```python
from build123d import *

# Parameters (mm, degrees)
SKETCH_1_W          = 40
SKETCH_1_H          = 14
EXTRUDE_1_DEPTH     = 40
SKETCH_6_W          = 36
SKETCH_6_H          = 10
CUT_EXTRUDE_2_DEPTH = 41
SKETCH_15_OUTSIDE_W = 53.656
SKETCH_15_OUTSIDE_H = 27.656
CUT_EXTRUDE_5_DEPTH = 41
SKETCH_16_W         = 50
SKETCH_16_H         = 24
EXTRUDE_2_DEPTH     = 1
SKETCH_17_W         = 50
SKETCH_17_H         = 24
EXTRUDE_3_DEPTH     = 1
SKETCH_18_W         = 36
SKETCH_18_H         = 10
CUT_EXTRUDE_6_DEPTH = 1


with BuildPart() as part:
    # 草图1 → 凸台-拉伸1 (new body)
    with BuildSketch(Plane(origin=(0, 0, 0), x_dir=(1, 0, 0), z_dir=(0, 1, 0))):
        with Locations((20, 7)):
            Rectangle(SKETCH_1_W, SKETCH_1_H)
    extrude(amount=EXTRUDE_1_DEPTH)

    # 草图6 → 切除-拉伸2 (cut, through all)
    with BuildSketch(Plane(origin=(0, 40, 0), x_dir=(1, 0, 0), z_dir=(0, 1, 0))):
        with Locations((20, 7)):
            Rectangle(SKETCH_6_W, SKETCH_6_H)
    extrude(amount=-CUT_EXTRUDE_2_DEPTH, mode=Mode.SUBTRACT)

    # 草图15 outside → 切除-拉伸5 (cut, through all)
    with BuildSketch(Plane.XZ):
        with Locations((20, -7)):
            Rectangle(SKETCH_15_OUTSIDE_W, SKETCH_15_OUTSIDE_H)
        with BuildLine():
            Line((2, -14), (38, -14))
            ThreePointArc((38, -14), (39.414213562, -13.414213562), (40, -12))
            Line((40, -12), (40, -2))
            ThreePointArc((40, -2), (39.414213562, -0.585786438), (38, 0))
            Line((38, 0), (2, 0))
            ThreePointArc((2, 0), (0.585786438, -0.585786438), (0, -2))
            Line((0, -2), (0, -12))
            ThreePointArc((0, -12), (0.585786438, -13.414213562), (2, -14))
        make_face(mode=Mode.SUBTRACT)
    extrude(amount=-CUT_EXTRUDE_5_DEPTH, mode=Mode.SUBTRACT)

    # 草图16 → 凸台-拉伸2 (add)
    with BuildSketch(Plane(origin=(0, 40, 0), x_dir=(1, 0, 0), z_dir=(0, 1, 0))):
        with Locations((20, 7)):
            Rectangle(SKETCH_16_W, SKETCH_16_H)
    extrude(amount=EXTRUDE_2_DEPTH)

    # 草图17 → 凸台-拉伸3 (add)
    with BuildSketch(Plane.XZ):
        with Locations((20, -7)):
            Rectangle(SKETCH_17_W, SKETCH_17_H)
    extrude(amount=EXTRUDE_3_DEPTH)

    # 草图18 → 切除-拉伸6 (cut)
    with BuildSketch(Plane(origin=(0, -1, 0), x_dir=(-1, 0, 0), z_dir=(0, -1, 0))):
        with Locations((-20, 7)):
            Rectangle(SKETCH_18_W, SKETCH_18_H)
    extrude(amount=-CUT_EXTRUDE_6_DEPTH, mode=Mode.SUBTRACT)


solid = part.part
```
Can you work these out from the model? Positions are in its coordinate system, mm. A direction names the side the tool comes from. Coordinates: 2 decimals unless noted, no trailing zeros. Loops run counter-clockwise (first coordinate to the right, second up) from the corner with the lowest first, then second, coordinate; pieces in that order, holes last. Notation, with made-up numbers: (53.25, 51.5) - (78.25, 51.5) arc R12 ccw to (78.25, 71.5) - close; hole circle Ø8 at (49, 6). An arc over 180 degrees is marked (long way). Use a Markdown table: item, result.
Item 1: I want a section at D-D on x = 29.5. Please give me the cut outline in (y, z).
Numbers:
| item | result |
|---|---|
| outline | (-1, -19) - (0, -19) - (0, -14) - (40, -14) - (40, -19) - (41, -19) - (41, 5) - (40, 5) - (40, 0) - (0, 0) - (0, 5) - (-1, 5) - (-1, -2) - (40, -2) - (40, -12) - (-1, -12) - close |
Item 2: I want a section at C-C on z = -10.5. Please give me the cut outline in (x, y).
Numbers:
| item | result |
|---|---|
| outline | (-5, -1) - (2, -1) - (2, 40) - (38, 40) - (38, -1) - (45, -1) - (45, 0) - (40, 0) - (40, 40) - (45, 40) - (45, 41) - (-5, 41) - (-5, 40) - (0, 40) - (0, 0) - (-5, 0) - close |
Item 3: I want a section at B-B on y = 33. Please give me the cut outline in (x, z).
Numbers:
| item | result |
|---|---|
| outline | (0, -12) arc R2 ccw to (2, -14) - (38, -14) arc R2 ccw to (40, -12) - (40, -2) arc R2 ccw to (38, 0) - (2, 0) arc R2 ccw to (0, -2) - close; hole (2, -12) - (38, -12) - (38, -2) - (2, -2) - close |
Item 4: We'd pull the mould along Z, two halves only. Please class faces 6 (the face through (0.57, 19.72, -13.4)), 7 (the face through (40, 20, -7)), 8 (the face through (38, 19, -7)): released by +Z, released by -Z, zero draft, split by the parting line, or undercut.
Numbers:
| item | result |
|---|---|
| face 6 | released by -Z |
| face 7 | zero draft |
| face 8 | undercut |
Item 5: For faces 1 (the face through (0.6, 19.72, -0.57)), 2 (the face through (39.4, 19.72, -13.43)), 3 (the face through (20, 19, -2)), 4 (the face through (0, 20, -7)), 5 (the face through (20, 20, 0)), which set-ups out of +Z, -Z, +X, -X, +Y, -Y let a thin tool reach every point of the face, with its end or its side?
Numbers:
| item | result |
|---|---|
| face 1 | +Z, -X |
| face 2 | -Z, +X |
| face 3 | -Y |
| face 4 | +Z, -Z, -X |
| face 5 | +Z, +X, -X |
Item 6: I want a section at A-A on z = -16.75. Please give me the cut outline in (x, y), and give its area (3 significant figures).
Numbers:
| item | result |
|---|---|
| outline | (-5, -1) - (45, -1) - (45, 0) - (-5, 0) - close; (-5, 40) - (45, 40) - (45, 41) - (-5, 41) - close |
| area | 100 mm2 |
Item 7: Will these pins go through, and if not, where does the flat tip stop? pin 1 (10 mm diameter, centred on x = 4, y = 21, fed in from -Z); pin 2 (8 mm diameter, centred on y = 21.5, z = -6.5, fed in from +X); pin 3 (6 mm diameter, centred on y = 12.5, z = -4.5, fed in from -X).
Numbers:
| item | result |
|---|---|
| pin 1 | stops at z = -14 |
| pin 2 | stops at x = 40 |
| pin 3 | stops at x = 0 |
Item 8: If I drill on probe 1 along Z at (x, y) = (8, 12.5); probe 2 along X at (y, z) = (21, -10.25); probe 3 along Y at (x, z) = (19.5, 4), over which ranges is the centre line in solid material (lowest first)? Write a range as from..to.
Numbers:
| item | result |
|---|---|
| probe 1 | z = -14..-12, -2..0 |
| probe 2 | x = 0..2, 38..40 |
| probe 3 | y = -1..0, 40..41 |
